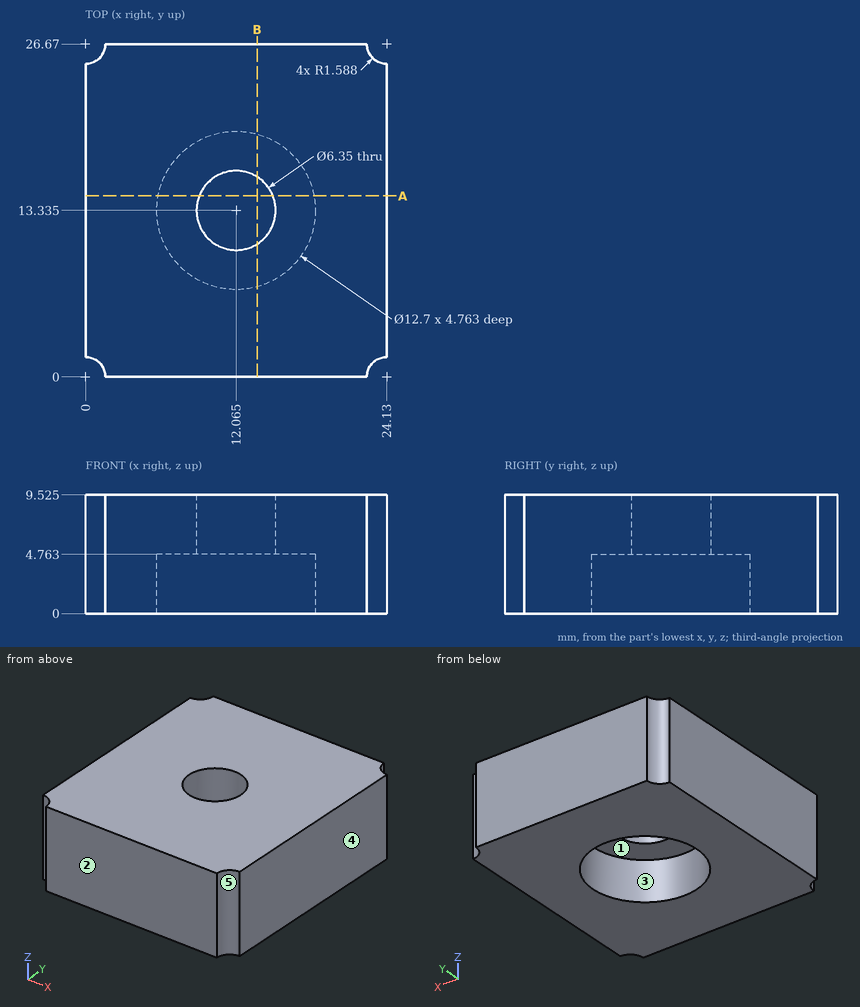
The figure shows three views and two pictorial views of one solid part (mm, origin at its lowest corner). Answer the questions. A direction names the side the tool comes from. Round coordinates to 2 decimals unless told otherwise and drop trailing zeros. Write each loop counter-clockwise with the first axis right and the second up, starting at its lowest first coordinate (ties: lowest second). Pieces come first, ordered by that corner, then holes. Notation, with made-up numbers: (43, -23.5) - (94, -23.5) arc R13 cw to (94, -18.5) - close; hole circle Ø2 at (66, -25). An arc over 180 degrees is marked (long way). Answer in a Markdown table with one row per item. Add a question column.
1. For the marked faces 1 and 2, determine the directions among +Z, -Z, +X, -X, +Y, -Y from which every point of the face is accessible in a straight line to the end or side of a thin tool.
2. Given pin 1 (3 mm diameter, centred on y = 15, z = 5.5, fed in from -X), flat-ended and moving along its own axis, determine where the tip first touches the part or whether it passes through.
3. A cutting plane is placed at A-A, the plane y = 14.5. Determine the outline of the cut face in (x, z) (1 decimal).
4. A cutting plane is placed at B-B, the plane x = 13.75. Determine the outline of the cut face in (y, z) (1 decimal), and give its area (3 significant figures).
5. Find the intervals of material crossed by line 1 along Z through (x, y) = (8.75, 14.75) (1 decimal); line 2 along X through (y, z) = (17.25, 2) (1 decimal); line 3 along X through (y, z) = (14.5, 2), in increasing order. Write a range as from..to.
6. The mould has two halves that part along Y. Classify the marked faces 3, 4 and 5: +Y half, -Y half, draft (parallel to the pull), parting line (faces both ways), or undercut.
Worked out:
| question | item | result |
|---|---|---|
| 1 | face 1 | -Z |
| 1 | face 2 | +Z, -Z, +X, -X, -Y |
| 2 | pin 1 | x = 0 |
| 3 | outline | (0, 0) - (5.8, 0) - (5.8, 4.8) - (9.1, 4.8) - (9.1, 9.5) - (0, 9.5) - close; (15, 4.8) - (18.3, 4.8) - (18.3, 0) - (24.1, 0) - (24.1, 9.5) - (15, 9.5) - close |
| 4 | outline | (0, 0) - (7.2, 0) - (7.2, 4.8) - (10.6, 4.8) - (10.6, 9.5) - (0, 9.5) - close; (16, 4.8) - (19.5, 4.8) - (19.5, 0) - (26.7, 0) - (26.7, 9.5) - (16, 9.5) - close |
| 4 | area | 170 mm^2 |
| 5 | line 1 | 4.8..9.5 |
| 5 | line 2 | 0..7.1, 17.1..24.1 |
| 5 | line 3 | 0..5.82, 18.31..24.13 |
| 6 | face 3 | undercut |
| 6 | face 4 | draft |
| 6 | face 5 | -Y half |
